from build123d import *

# Parameters (mm, degrees)
F1_DEPTH = 50.8


with BuildPart() as f1:
    # F0 (on Top) → F1 (new body)
    with BuildSketch(Plane.XY):
        with BuildLine():
            Line((-34.573272, 22.455608), (-43.223512, 7.902216))
            ThreePointArc((-43.223512, 7.902216), (-44.954669, 0.268443), (-41.880949, -6.93042))
            Line((-41.880949, -6.93042), (-34.677799, -15.196177))
            ThreePointArc((-34.677799, -15.196177), (-30.362733, -18.412203), (-25.103225, -19.552464))
            Line((-25.103225, -19.552464), (20.536096, -19.552464))
            ThreePointArc((20.536096, -19.552464), (24.833093, -18.80344), (28.623231, -16.644718))
            Line((28.623231, -16.644718), (38.985124, -8.087135))
            ThreePointArc((38.985124, -8.087135), (43.540626, 0.499418), (40.690243, 9.792254))
            Line((40.690243, 9.792254), (28.912036, 24.05382))
            ThreePointArc((28.912036, 24.05382), (24.531961, 27.455736), (19.119781, 28.666684))
            Line((19.119781, 28.666684), (-23.656136, 28.666684))
            ThreePointArc((-23.656136, 28.666684), (-29.93629, 27.005238), (-34.573272, 22.455608))
        make_face()
    extrude(amount=F1_DEPTH)


solid = f1.part
Work out the finished part from the listing and answer in its coordinate system (mm). Coordinates: 2 decimals unless noted, no trailing zeros. Write each loop counter-clockwise with the first axis right and the second up, starting at its lowest first coordinate (ties: lowest second). Pieces come first, ordered by that corner, then holes. Notation, with made-up numbers: M 33,-13 L 92,-13 A24 cw 92,11 Z; hole C 8.5,-10 d8. An arc over 180 degrees is marked long. Write item = value, one per line.
1. The part is cut by section C-C (y = -13). Determine the outline of the cut face in (x, z), then the cut area to 3 significant figures.
Solution:
outline = M -36.59,0 L 33.04,0 L 33.04,50.8 L -36.59,50.8 Z
area = 3,540 mm2
2. Straight lines are drawn through the part: line 1 (Y direction, x = -33.5, z = 3); line 2 (X direction, y = 3, z = 2.5); line 3 (Y direction, x = -36.5, z = 29). For each, find the intervals that lie inside material, in ascending order. Write a range as from..to.
Solution:
line_1 = -16.38..23.99
line_2 = -44.91..43.53
line_3 = -13.11..19.21
3. The part is cut by section A-A (z = 22). Determine the outline of the cut face in (x, y).
Solution:
outline = M -43.22,7.9 A12.7 ccw -41.88,-6.93 L -34.68,-15.2 A12.7 ccw -25.1,-19.55 L 20.54,-19.55 A12.7 ccw 28.62,-16.64 L 38.99,-8.09 A12.7 ccw 40.69,9.79 L 28.91,24.05 A12.7 ccw 19.12,28.67 L -23.66,28.67 A12.7 ccw -34.57,22.46 Z
4. Flat-ended cylindrical pins translate along their axes: pin 1 (2 mm diameter, centred on x = -26.5, z = 36.5, fed in from -Y); pin 2 (8 mm diameter, centred on y = -13, z = 33.5, fed in from +X); pin 3 (5 mm diameter, centred on y = -5, z = 11.5, fed in from +X). Find the tip coordinate at first contact, or state that the pin passes through.
Solution:
pin_1 = -19.55
pin_2 = 37.88
pin_3 = 42.88
5. The part is cut by section B-B (y = 12.5). Determine the outline of the cut face in (x, z).
Solution:
outline = M -40.49,0 L 38.45,0 L 38.45,50.8 L -40.49,50.8 Z
